Study the drawing (mm; zero at the part's minimum x, y, z) and answer. A direction names the side the tool comes from. Give positions to 0.01 mm unless a question says otherwise; leave off trailing zeros. Loops run counter-clockwise (first coordinate to the right, second up) from the corner with the lowest first, then second, coordinate; pieces in that order, holes last. Notation, with made-up numbers: M -9.75,17 L 3.25,17 A21 cw 3.25,55 Z; hole C 39,55.5 d11. An arc over 180 degrees is marked long. Return JSON: item names as keys, results as strings.
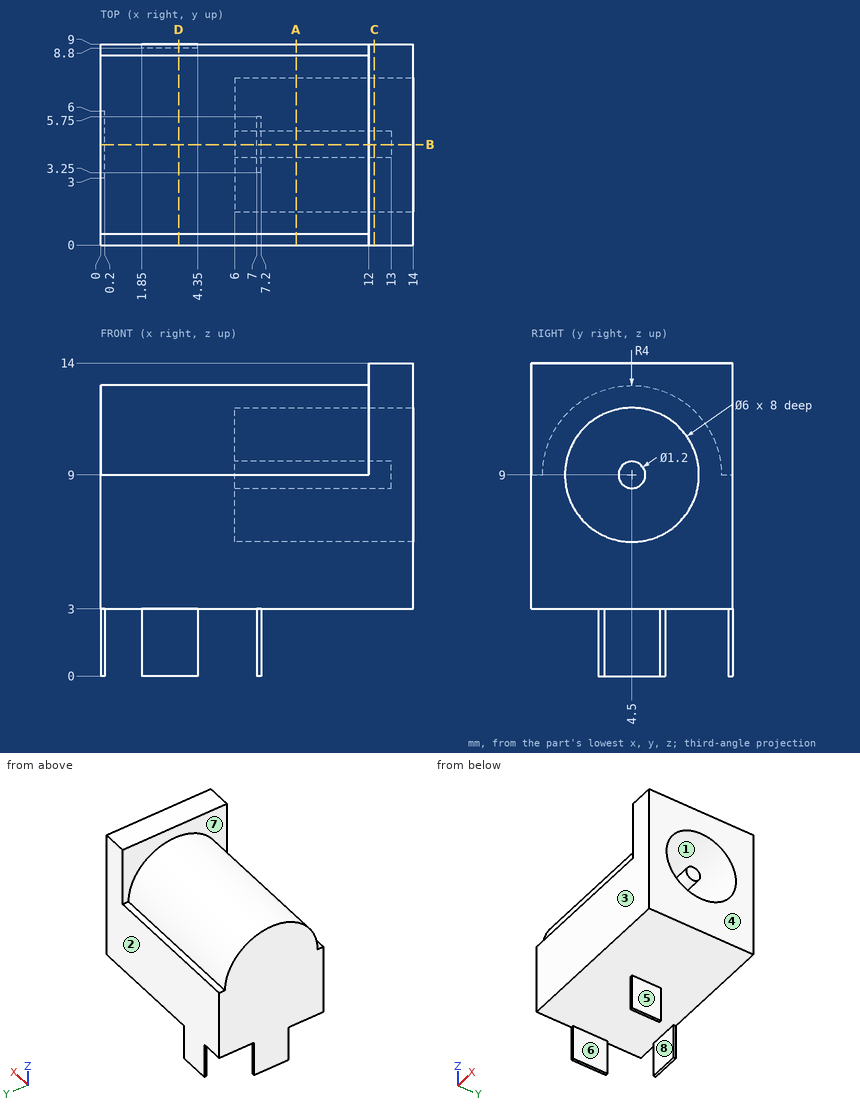
(1) The part is cut by section D-D (x = 3.5). Determine the outline of the cut face in (y, z).
Values follow:
{"outline": "M 0,3 L 8.8,3 L 8.8,0 L 9,0 L 9,9 L 8.5,9 A4 ccw 0.5,9 L 0,9 Z"}
(2) Straight lines are drawn through the part: line 1 along Y through (x, z) = (12.5, 9); line 2 along Z through (x, y) = (10, 5); line 3 along X through (y, z) = (4.25, 1.25). For each, find the intervals that lie inside material, in ascending order.
Values follow:
{"line 1": "0 to 1.5, 3.9 to 5.1, 7.5 to 9", "line 2": "3 to 6.04, 8.67 to 9.33, 11.96 to 12.97", "line 3": "0 to 0.2, 7 to 7.2"}
(3) A tool of negligible diameter and unlimited length cuts with its end or side. For the marked faces 5, 6, 7 and 8, from which of +Z, -Z, +X, -X, +Y, -Y can it reach the whole face along a straight path? Write none if from no direction.
Values follow:
{"face 5": "-Z, +X, +Y, -Y", "face 6": "-Z, +Y, -Y", "face 7": "+Z, -X", "face 8": "-Z, +X, -X, -Y"}
(4) Determine the mould class of the marked faces 1, 2, 3 and 4 for opening direction Y: released by +Y, released by -Y, zero draft, split by the parting line, or undercut.
Values follow:
{"face 1": "undercut", "face 2": "released by +Y", "face 3": "released by -Y", "face 4": "zero draft"}
(5) The part is cut by section C-C (x = 12.25). Determine the outline of the cut face in (y, z), and give its area (3 significant figures).
Values follow:
{"outline": "M 0,3 L 9,3 L 9,14 L 0,14 Z; C 4.5,9 d1.2; hole C 4.5,9 d6", "area": "71.9 mm²"}
(6) Given pin 1 (1 mm diameter, centred on y = 4, z = 8.5, fed in from +X); pin 2 (4 mm diameter, centred on x = 2, y = 7.5, fed in from +Z); pin 3 (0.8 mm diameter, centred on y = 4.5, z = 2, fed in from +X), each flat-ended and moving along its own axis, determine where each tip first touches the part or whether it passes through.
Values follow:
{"pin 1": "x = 13", "pin 2": "z = 12.87", "pin 3": "x = 7.2"}
(7) The part is cut by section A-A (x = 8.75). Determine the outline of the cut face in (y, z).
Values follow:
{"outline": "M 0,3 L 9,3 L 9,9 L 8.5,9 A4 ccw 0.5,9 L 0,9 Z; C 4.5,9 d1.2; hole C 4.5,9 d6"}
(8) The part is cut by section B-B (y = 4.5). Determine the outline of the cut face in (x, z).
Values follow:
{"outline": "M 0,0 L 0.2,0 L 0.2,3 L 7,3 L 7,0 L 7.2,0 L 7.2,3 L 14,3 L 14,6 L 6,6 L 6,8.4 L 13,8.4 L 13,9.6 L 6,9.6 L 6,12 L 14,12 L 14,14 L 12,14 L 12,13 L 0,13 Z"}
